Verification items for the finished model (mm, model axes). A direction names the side the tool comes from. Round coordinates to 2 decimals unless told otherwise and drop trailing zeros. Loops run counter-clockwise (first coordinate to the right, second up) from the corner with the lowest first, then second, coordinate; pieces in that order, holes last. Notation, with made-up numbers: (65.25, 36) - (111.25, 36) arc R28 ccw to (111.25, 74) - close; hole circle Ø5 at (22, 29). An arc over 180 degrees is marked (long way). Use a Markdown table: item, result. Add a question column.
```python
from build123d import *

# Parameters (mm, degrees)
CORTAR_EXTRUIR1_DEPTH = 10


with BuildPart() as part:
    # Croquis1 → Revolución1 (revolve)
    with BuildSketch(Plane.XY, mode=Mode.PRIVATE) as revoluci_n1_sk:
        Polygon((-17.904415608, -1.515813334), (-17.904415608, 2.284186666), (-18.904415608, 2.284186666), (-18.904415608, -0.515813334), (-25.304415608, -0.515813334), (-25.304415608, 2.284186666), (-26.304415608, 2.284186666), (-26.304415608, -1.515813334), align=None)
    revolve(revoluci_n1_sk.sketch.rotate(Axis((-16.004415608, 9.150344382, 0), (0, -1, 0)), 270), axis=Axis((-16.004415608, 9.150344382, 0), (0, -1, 0)))

    # Croquis2 → Cortar-Extruir1 (cut)
    with BuildSketch(Plane(origin=(0, 2.284186666, 0), x_dir=(1, 0, 0), z_dir=(0, 1, 0))):
        with BuildLine():
            Line((-17.904415608, 0), (-24.175391996, -6.270976388))
            ThreePointArc((-24.175391996, -6.270976388), (-16.004415608, -10.3), (-7.833439219, -6.270976388))
            Line((-7.833439219, -6.270976388), (-14.104415608, 0))
            ThreePointArc((-14.104415608, 0), (-16.004415608, -1.9), (-17.904415608, 0))
        make_face()
    extrude(amount=-CORTAR_EXTRUIR1_DEPTH, mode=Mode.SUBTRACT)


solid = part.part
```
Q1. Section check B-B on y = 0. Record the cut outline in (x, z), plus the area to 3 significant figures.
Q2. Go/stop test with flat-tipped pins: pin 1 Ø2 at (x, y) = (-24, 1) entering from -Z; pin 2 Ø1 at (x, y) = (-8.5, 0.5) entering from +Z. Record where each tip stops, or that it passes through.
Q3. Thickness scan on line 1 along X through (y, z) = (0, -1.25); line 2 along X through (y, z) = (0.95, -0.25); line 3 along Y through (x, z) = (-19.75, -6.25). Record the ranges inside material, lowest first.
Q4. Section check C-C on x = -24.5. Record the cut outline in (y, z).
Q5. Section check A-A on z = 0.5. Record the cut outline in (x, y), plus the area to 3 significant figures.
Q6. Section check D-D on z = 3.5. Record the cut outline in (x, y), plus the area to 3 significant figures.
Q7. Release check for a two-part mould opening along Z. For faces 4 (the face through (-16.1, -0.516, -3.4)), 5 (the face through (-16.325, 0.358, -10.295)), 6 (the face through (-16.1, -1.516, -2.1)) record: +Z half, -Z half, draft (parallel to the pull), parting line (faces both ways), or undercut.
Q8. Set-up check for faces 1 (the face through (-17.58, 2.284, -9.34)), 2 (the face through (-16.1, 0.9, -2.9)), 3 (the face through (-10.925, -0.856, 3.179)): record each of +Z, -Z, +X, -X, +Y, -Y from which the full face is reachable in a straight line by a thin tool's end or side.
Determined:
| question | item | result |
|---|---|---|
| 1 | outline | (-24.18, 6.27) arc R10.3 ccw (long way) to (-7.83, 6.27) - (-8.55, 5.56) arc R9.3 cw (long way) to (-23.46, 5.56) - close; (-18.77, 0.87) arc R2.9 ccw (long way) to (-13.24, 0.87) - (-14.1, 0) arc R1.9 cw to (-17.9, 0) - close |
| 1 | area | 51.9 mm² |
| 2 | pin 1 | stops at z = -7.56 |
| 2 | pin 2 | stops at z = 6.1 |
| 3 | line 1 | x = -26.23 to -25.22, -18.62 to -17.44, -14.57 to -13.39, -6.79 to -5.78 |
| 3 | line 2 | x = -26.3 to -25.3, -18.89 to -17.89, -14.12 to -13.12, -6.71 to -5.71 |
| 3 | line 3 | y = -1.52 to -0.52 |
| 4 | outline | (-1.52, -5.82) - (2.28, -5.82) - (2.28, -3.78) - (-0.52, -3.78) - (-0.52, 3.78) - (2.28, 3.78) - (2.28, 5.82) - (-1.52, 5.82) - close |
| 5 | outline | (-26.29, -1.52) - (-18.4, -1.52) - (-18.4, 2.28) - (-18.86, 2.28) - (-18.86, -0.52) - (-25.29, -0.52) - (-25.29, 2.28) - (-26.29, 2.28) - close; (-13.6, -1.52) - (-5.72, -1.52) - (-5.72, 2.28) - (-6.72, 2.28) - (-6.72, -0.52) - (-13.15, -0.52) - (-13.15, 2.28) - (-13.6, 2.28) - close |
| 5 | area | 23.9 mm² |
| 6 | outline | (-25.69, -1.52) - (-21.4, -1.52) - (-21.4, -0.52) - (-24.62, -0.52) - (-24.62, 2.28) - (-25.69, 2.28) - close; (-10.6, -1.52) - (-6.32, -1.52) - (-6.32, 2.28) - (-7.39, 2.28) - (-7.39, -0.52) - (-10.6, -0.52) - close |
| 6 | area | 14.6 mm² |
| 7 | face 4 | undercut |
| 7 | face 5 | parting line |
| 7 | face 6 | draft |
| 8 | face 1 | +Z, -Z, +X, -X, +Y |
| 8 | face 2 | +Y |
| 8 | face 3 | +Z, +Y, -Y |
